```python
from build123d import *

# Parameters (mm, degrees)
F1_DEPTH  = 14
F2_R      = 2.75
F3_DEPTH  = 1
F4_R      = 1.5
F5_DEPTH  = 6.75
F6_R      = 1
F7_DEPTH  = 15
F9_DEPTH  = 8
F10_R     = 1.5
F11_DEPTH = 12
F12_SIZE  = 2


with BuildPart() as f1:
    # F0 (on Top) → F1 (new body)
    with BuildSketch(Plane.XY):
        with BuildLine():
            Line((-72.3968957005, -4.1161350385), (-112.3968957005, -4.1161350385))
            ThreePointArc((-112.3968957005, -4.1161350385), (-141.4063263067, -12.6161350385), (-112.3968957005, -21.1161350385))
            Line((-112.3968957005, -21.1161350385), (-97.3968957005, -21.1161350385))
            Line((-97.3968957005, -21.1161350385), (-97.3968957005, -13.3661350385))
            Line((-97.3968957005, -13.3661350385), (-117.2151498361, -13.3661350385))
            ThreePointArc((-117.2151498361, -13.3661350385), (-134.1563263067, -12.6161350385), (-117.2151498361, -11.8661350385))
            Line((-117.2151498361, -11.8661350385), (-95.9651498361, -11.8661350385))
            Line((-95.9651498361, -11.8661350385), (-95.9651498361, -21.1161350385))
            Line((-95.9651498361, -21.1161350385), (-72.3968957005, -21.1161350385))
            Line((-72.3968957005, -21.1161350385), (-72.3968957005, -4.1161350385))
        make_face()
    extrude(amount=F1_DEPTH)

    # F2 (on face) → F3 (cut)
    with BuildSketch(Plane.XZ.offset(21.1161350386)):
        with Locations((-104.8968957005, 7)):
            Circle(F2_R)
    extrude(amount=-F3_DEPTH, mode=Mode.SUBTRACT)

    # F4 (on face) → F5 (cut, through all)
    with BuildSketch(Plane.XZ.offset(20.1161350386)):
        with Locations((-104.8968957005, 7)):
            Circle(F4_R)
    extrude(amount=-F5_DEPTH, mode=Mode.SUBTRACT)

    # F6 (on face) → F7 (cut)
    with BuildSketch(Plane.XZ.offset(20.1161350386)):
        with Locations((-104.8968957005, 7)):
            Circle(F6_R)
    extrude(amount=-F7_DEPTH, mode=Mode.SUBTRACT)

    # F8 (on face) → F9 (cut)
    with BuildSketch(Plane(origin=(0, 0, 0), x_dir=(1, 0, 0), z_dir=(0, 0, -1))):
        with BuildLine():
            ThreePointArc((-109.9262055214, 13.3661350385), (-110.6529561162, 17.403274319), (-112.3968957005, 21.1161350385))
            ThreePointArc((-112.3968957005, 21.1161350385), (-141.4063263067, 12.6161350385), (-112.3968957005, 4.1161350385))
            ThreePointArc((-112.3968957005, 4.1161350385), (-110.6529561162, 7.8289957581), (-109.9262055214, 11.8661350385))
            Line((-109.9262055214, 11.8661350385), (-117.2151498361, 11.8661350385))
            ThreePointArc((-117.2151498361, 11.8661350385), (-134.1563263067, 12.6161350385), (-117.2151498361, 13.3661350385))
            Line((-117.2151498361, 13.3661350385), (-109.9262055214, 13.3661350385))
        make_face()
    extrude(amount=-F9_DEPTH, mode=Mode.SUBTRACT)

    # F10 (on face) → F11 (cut)
    with BuildSketch(Plane(origin=(0, 0, 0), x_dir=(1, 0, 0), z_dir=(0, 0, -1))):
        with Locations((-79.6468957005, 12.6161350385)):
            Circle(F10_R)
        with Locations((-86.8968957005, 12.6161350385)):
            Circle(F10_R)
    extrude(amount=-F11_DEPTH, mode=Mode.SUBTRACT)

    # F12
    f12_edges = [f1.edges().sort_by_distance(p)[0] for p in [
        (-72.396896, -4.116135, 7),
        (-72.396896, -21.116135, 7),
    ]]
    chamfer(f12_edges, length=F12_SIZE)


solid = f1.part
```
Design review of the part built by this model. Coordinates are the model's own, in mm. A direction names the side the tool comes from. Coordinates: 2 decimals unless noted, no trailing zeros. Write each loop counter-clockwise with the first axis right and the second up, starting at its lowest first coordinate (ties: lowest second). Pieces come first, ordered by that corner, then holes.
1) Add section B-B (x = -100). Write out the cut boundary in (y, z).
2) Add section D-D (x = -124). Write out the cut boundary in (y, z).
3) Add section A-A (y = -9.5). Write out the cut boundary in (x, z), plus the area to 3 significant figures.
4) To check wall thickness, follow L1, parallel to Y at x = -102.5, z = 12; L2, parallel to X at y = -20, z = 6.5; L3, parallel to Y at x = -87, z = 5.75. State the ranges of each line that lie inside material, in increasing order.
5) Mouldability with a two-part tool opening along Y and no side actions: class faces 1 (the flat face through (-103.7, -20.116, 5.8)), 2 (the flat face through (-95.965, -16, 7)), 3 (the cylindrical face through (-110.636, -17.348, 3.944)), 4 (the flat face through (-104, -11.866, 8)) as +Y half, -Y half, draft (parallel to the pull), parting line (faces both ways), or undercut.
6) Insertion check: pin 1 (3 mm diameter, centred on y = -18, z = 9.5, fed in from -X); pin 2 (3.5 mm diameter, centred on x = -79.5, y = -12, fed in from -Z); pin 3 (4 mm diameter, centred on x = -83.5, z = 5.5, fed in from -Y); pin 4 (12 mm diameter, centred on x = -124.5, y = -1, fed in from -Z). Each pin has a flat end and moves straight along its axis. Give the tip position at first contact, or say it passes through.
7) Machinability: for faces 5 (the cylindrical face through (-110.67, -7.77, 3.94)), 6 (the cylindrical face through (-106.09, -16.79, 6.09)), 7 (the flat face through (-97.397, -17, 7)), 8 (the cylindrical face through (-78.216, -13.067, 5.916)), 9 (the flat face through (-93, -4.116, 7)), which of the approach directions +Z, -Z, +X, -X, +Y, -Y give a long, thin tool a straight path to every point of the face, cutting with its end or side? Answer none if there is none.
8) Add section C-C (z = 7). Write out the cut boundary in (x, y), plus the area to 3 significant figures.
Check result:
1. outline: (-21.12, 0) - (-13.37, 0) - (-13.37, 14) - (-21.12, 14) - close; (-11.87, 0) - (-4.12, 0) - (-4.12, 14) - (-11.87, 14) - close
2. outline: (-28.28, 8) - (-20.94, 8) - (-20.94, 14) - (-28.28, 14) - close; (-4.29, 8) - (3.05, 8) - (3.05, 14) - (-4.29, 14) - close
3. outline: (-141.09, 8) - (-133.56, 8) - (-133.56, 14) - (-141.09, 14) - close; (-117.77, 8) - (-110.22, 8) - (-110.22, 0) - (-72.4, 0) - (-72.4, 14) - (-117.77, 14) - close; hole circle Ø2 at (-104.9, 7)
3. area: 617 mm2
4. L1: y = -21.12 to -13.37, -11.87 to -4.12
4. L2: x = -111.75 to -106.31, -103.48 to -97.4, -95.97 to -73.28
4. L3: y = -21.12 to -14.11, -11.12 to -4.12
5. face 1: -Y half
5. face 2: draft
5. face 3: undercut
5. face 4: undercut
6. pin 1: stops at x = -140.92
6. pin 2: stops at z = 0
6. pin 3: stops at y = -21.12
6. pin 4: stops at z = 8
7. face 5: -Z, -X
7. face 6: -Y
7. face 7: +Z, -Z, -Y
7. face 8: -Z
7. face 9: +Z, -Z, +X, +Y
8. outline: (-112.4, -21.12) - (-107.65, -21.12) - (-107.65, -20.12) - (-106.4, -20.12) - (-106.4, -13.37) - (-109.93, -13.37) arc R15.76 cw to start; (-112.4, -4.12) arc R15.76 cw to (-109.93, -11.87) - (-105.9, -11.87) - (-105.9, -5.12) - (-103.9, -5.12) - (-103.9, -11.87) - (-95.97, -11.87) - (-95.97, -21.12) - (-74.4, -21.12) - (-72.4, -19.12) - (-72.4, -6.12) - (-74.4, -4.12) - close; (-103.4, -20.12) - (-102.15, -20.12) - (-102.15, -21.12) - (-97.4, -21.12) - (-97.4, -13.37) - (-103.4, -13.37) - close; hole circle Ø3 at (-86.9, -12.62); hole circle Ø3 at (-79.65, -12.62)
8. area: 562 mm2
